Verification items for this drawing (mm, ordinates from the low corner). Give positions to 0.01 mm unless a question says otherwise; leave off trailing zeros. Write each loop counter-clockwise with the first axis right and the second up, starting at its lowest first coordinate (ties: lowest second). Pieces come first, ordered by that corner, then holes. Notation, with made-up numbers: (28, 47.5) -> (72, 47.5) arc R19 cw to (72, 77.5) -> close; hole circle Ø9 at (-12, 46.5). An arc over 180 degrees is marked (long way). Use one line per item in the form item = value. Start each with the question number.
(1) Section check A-A, the plane y = 1.25. Record the cut outline in (x, z) (1 decimal).
(2) Section check C-C, the plane x = 2.5. Record the cut outline in (y, z), plus the area to 3 significant figures.
(3) Scan lines: L1, parallel to X at y = 0.6, z = 18 (1 decimal); L2, parallel to Z at x = 3, y = 1.85; L3, parallel to X at y = 0.7, z = 37. Record each from-to range of solid material in increasing order.
(4) Section check B-B, the plane z = 27. Record the cut outline in (x, y) (1 decimal).
(5) Depth check by flat-ended pin: pin 1 Ø1 at (y, z) = (1.5, 26) entering from +X; pin 2 Ø0.6 at (y, z) = (1, 21.5) entering from -X. Enter the tip coordinate at first touch or a pass-through.
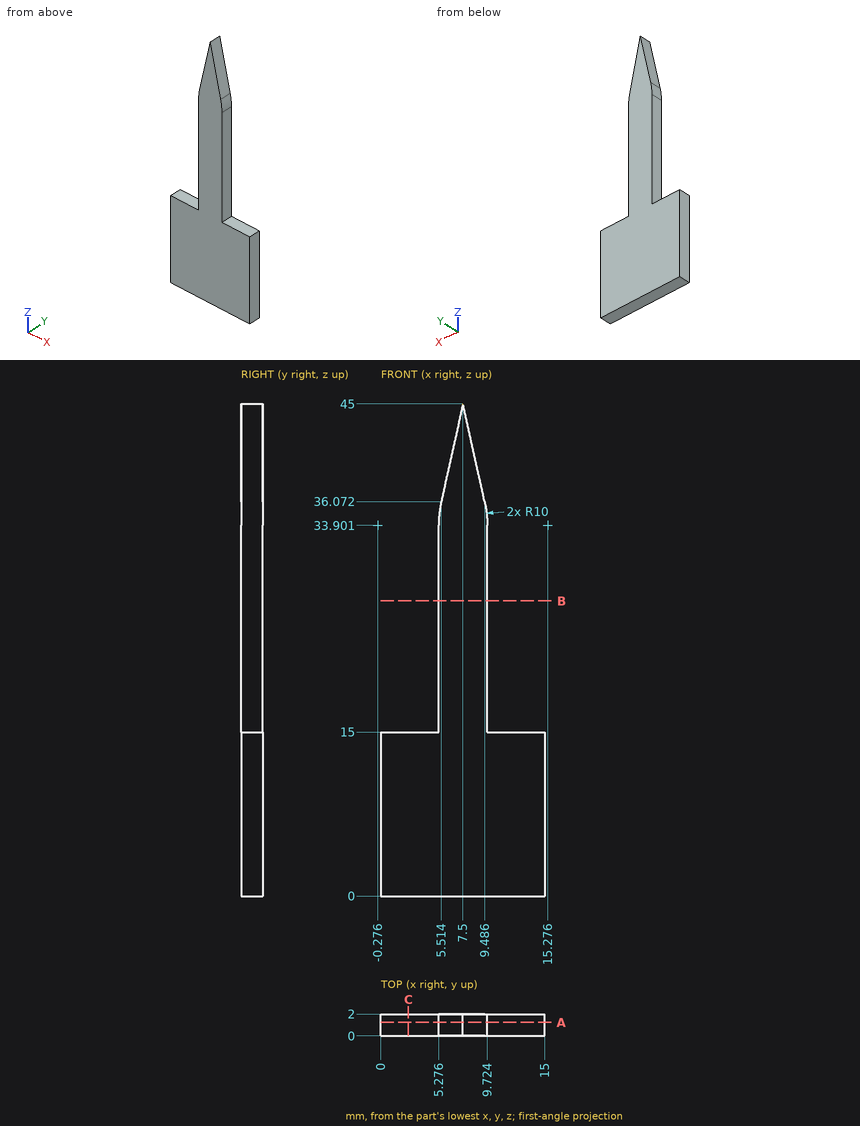
Completed:
q1.outline = (0, 0) -> (15, 0) -> (15, 15) -> (9.7, 15) -> (9.7, 33.9) arc R10 ccw to (9.5, 36.1) -> (7.5, 45) -> (5.5, 36.1) arc R10 ccw to (5.3, 33.9) -> (5.3, 15) -> (0, 15) -> close
q2.outline = (0, 0) -> (2, 0) -> (2, 15) -> (0, 15) -> close
q2.area = 30.0 mm²
q3.L1 = 5.3 to 9.7
q3.L2 = 0 to 15
q3.L3 = 5.72 to 9.28
q4.outline = (5.3, 0) -> (9.7, 0) -> (9.7, 2) -> (5.3, 2) -> close
q5.pin_1 = 9.72
q5.pin_2 = 5.28
